Answer from the drawing. Dimensions are ordinates in mm from the lowest x, y and z of the part. Coordinates: 2 decimals unless noted, no trailing zeros. Write each loop counter-clockwise with the first axis right and the second up, starting at its lowest first coordinate (ties: lowest second). Pieces come first, ordered by that corner, then holes. Notation, with made-up numbers: (70, 10) - (89, 10) arc R22 ccw to (89, 26) - close; hole circle Ø11 at (8, -34.5). An arc over 180 degrees is marked (long way). Use one line per item in the form item = value. Start each with the question number.
Item 1: A cutting plane is placed at B-B (z = 8). Write down the section's boundary in (x, y), then the cut area to 3 significant figures.
Item 2: Consider probe 1 along Z at (x, y) = (7.5, 3.25); probe 2 along X at (y, z) = (9.75, 3.25); probe 3 along Z at (x, y) = (5, 11.75). Determine where each line is inside the solid, lowest interval first.
Item 3: A cutting plane is placed at A-A (y = 6). Write down the section's boundary in (x, z).
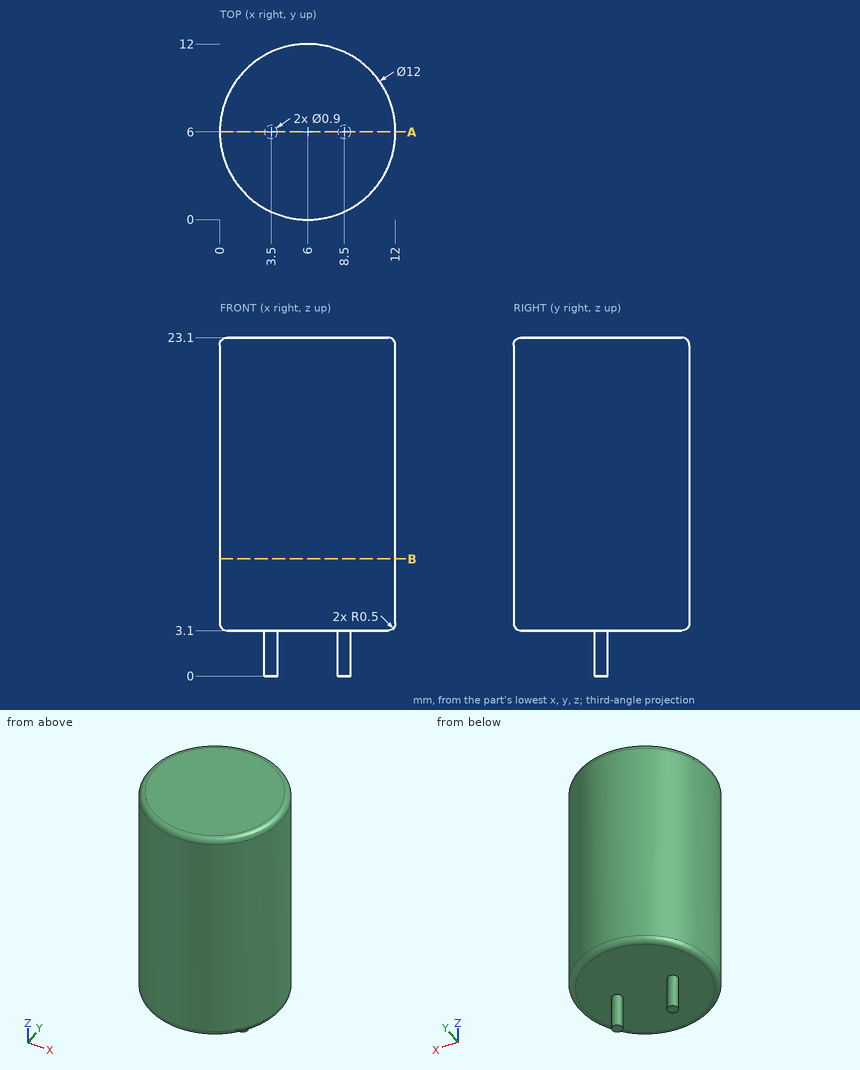
Answer:
q1.outline = circle Ø12 at (6, 6)
q1.area = 113 mm²
q2.probe_1 = 3.1 to 23.1
q2.probe_2 = 1.5 to 10.5
q2.probe_3 = 3.23 to 22.97
q3.outline = (0, 3.6) arc R0.5 ccw to (0.5, 3.1) - (3.05, 3.1) - (3.05, 0) - (3.95, 0) - (3.95, 3.1) - (8.05, 3.1) - (8.05, 0) - (8.95, 0) - (8.95, 3.1) - (11.5, 3.1) arc R0.5 ccw to (12, 3.6) - (12, 22.6) arc R0.5 ccw to (11.5, 23.1) - (0.5, 23.1) arc R0.5 ccw to (0, 22.6) - close
